Verification items for the finished model (mm, model axes). Face numbers are marked on the shaded views. A direction names the side the tool comes from. Give positions to 0.01 mm unless a question says otherwise; leave off trailing zeros. Loops run counter-clockwise (first coordinate to the right, second up) from the corner with the lowest first, then second, coordinate; pieces in that order, holes last. Notation, with made-up numbers: (68.25, 28) -> (107.25, 28) arc R10 cw to (107.25, 38) -> close; hole circle Ø10 at (-13, 18). An arc over 180 degrees is marked (long way). Answer in a Markdown table with one row per item. Add a question column.
Q1. Release check for a two-part mould opening along Z. For the marked faces 1, 2 and 3 record: pulls with the +Z half, pulls with the -Z half, needs draft (parallel to the pull), parting line crosses it, or undercut.
Q2. Section check D-D on z = -15.5. Enter the section's corners in (x, y).
Q3. Set-up check for the marked faces 4, 5 and 6: record each of +Z, -Z, +X, -X, +Y, -Y from which the full face is reachable in a straight line by a thin tool's end or side.
Q4. Material ranges on probe 1 along X at (y, z) = (7.65, 16); probe 2 along X at (y, z) = (2.5, 16.5), recorded low to high.
Q5. Section check C-C on x = -4. Enter the section's corners in (y, z), and give its area (3 significant figures).
Q6. Section check A-A on y = 8.75. Give the number of separate pieces and of enclosed holes in the cut face, and give its area (3 significant figures).
Q7. Gauge pin test, flat ends, axial feed: P1, Ø0.8, axis at x = 19.5, y = 7.5, coming from the -Z side; P2, Ø0.9, axis at y = 7, z = -15, coming from the -X side; P3, Ø0.8, axis at x = 9.5, y = 2.5, coming from the +Z side. Record the tip position at first contact, or that the pin passes through.
```python
from build123d import *

# Parameters (mm, degrees)
SKETCH1_W           = 40
SKETCH1_H           = 40
BOSS_EXTRUDE1_DEPTH = 5
SKETCH3_R           = 1
BOSS_EXTRUDE3_DEPTH = 5
SKETCH3_4_R         = 1
CUT_EXTRUDE1_DEPTH  = 5
SKETCH4_R           = 1
CUT_EXTRUDE2_DEPTH  = 10
CIRPATTERN2_COUNT   = 4


with BuildPart() as part:
    # Sketch1 → Boss-Extrude1 (new body)
    with BuildSketch(Plane(origin=(0, 0, 0), x_dir=(1, 0, 0), z_dir=(0, 1, 0))):
        Rectangle(SKETCH1_W, SKETCH1_H)
    extrude(amount=BOSS_EXTRUDE1_DEPTH)

    # Sketch3 → Boss-Extrude3 (add)
    # profile 1 of 4: a face of its own
    with BuildSketch(Plane(origin=(0, 5, 0), x_dir=(1, 0, 0), z_dir=(0, 1, 0))):
        with BuildLine():
            Line((11, 11), (18, 11))
            Line((18, 11), (18, 4))
            Line((18, 4), (20, 4))
            Line((20, 4), (20, 13))
            Line((20, 13), (19, 13))
            Line((19, 13), (19, 16))
            ThreePointArc((19, 16), (16, 19), (13, 16))
            Line((13, 16), (13, 13))
            Line((13, 13), (11, 13))
            Line((11, 13), (11, 11))
        make_face()
        with Locations(Location((16, 16, 0), (0, 0, 270))):
            Circle(SKETCH3_R, mode=Mode.SUBTRACT)
    # profile 2 of 4: a face of its own
    with BuildSketch(Plane(origin=(0, 5, 0), x_dir=(1, 0, 0), z_dir=(0, 1, 0))):
        with BuildLine():
            Line((-18, 11), (-11, 11))
            Line((-11, 11), (-11, 13))
            Line((-11, 13), (-13, 13))
            Line((-13, 13), (-13, 16))
            ThreePointArc((-13, 16), (-16, 19), (-19, 16))
            Line((-19, 16), (-19, 13))
            Line((-19, 13), (-20, 13))
            Line((-20, 13), (-20, 9))
            Line((-20, 9), (-18, 9))
            Line((-18, 9), (-18, 11))
        make_face()
        with BuildLine():
            ThreePointArc((-17, 16), (-16, 17), (-15, 16))
            Line((-15, 16), (-17, 16))
        make_face(mode=Mode.SUBTRACT)
    # profile 3 of 4: a face of its own
    with BuildSketch(Plane(origin=(0, 5, 0), x_dir=(1, 0, 0), z_dir=(0, 1, 0))):
        with BuildLine():
            Line((20, -4), (18, -4))
            Line((18, -4), (18, -11))
            Line((18, -11), (11, -11))
            Line((11, -11), (11, -13))
            Line((11, -13), (13, -13))
            Line((13, -13), (13, -16))
            ThreePointArc((13, -16), (16, -19), (19, -16))
            Line((19, -16), (19, -13))
            Line((19, -13), (20, -13))
            Line((20, -13), (20, -4))
        make_face()
    # profile 4 of 4: a face of its own
    with BuildSketch(Plane(origin=(0, 5, 0), x_dir=(1, 0, 0), z_dir=(0, 1, 0))):
        with BuildLine():
            Line((-11, -13), (-11, -11))
            Line((-11, -11), (-18, -11))
            Line((-18, -11), (-18, -9))
            Line((-18, -9), (-20, -9))
            Line((-20, -9), (-20, -13))
            Line((-20, -13), (-19, -13))
            Line((-19, -13), (-19, -16))
            ThreePointArc((-19, -16), (-16, -19), (-13, -16))
            Line((-13, -16), (-13, -13))
            Line((-13, -13), (-11, -13))
        make_face()
        with BuildLine():
            ThreePointArc((-15, -16), (-16, -17), (-17, -16))
            Line((-17, -16), (-15, -16))
        make_face(mode=Mode.SUBTRACT)
    extrude(amount=BOSS_EXTRUDE3_DEPTH)

    # Sketch3_4 → Cut-Extrude1 (cut)
    with BuildSketch(Plane(origin=(0, 5, 0), x_dir=(1, 0, 0), z_dir=(0, 1, 0))):
        with Locations(Location((-16, 16, 0), (0, 0, 270))):
            Circle(SKETCH3_4_R)
        with Locations(Location((-16, -16, 0), (0, 0, 270))):
            Circle(SKETCH3_4_R)
        with Locations(Location((16, -16, 0), (0, 0, 270))):
            Circle(SKETCH3_4_R)
    extrude(amount=CUT_EXTRUDE1_DEPTH, mode=Mode.SUBTRACT)

    # Sketch4 → Cut-Extrude2 (cut)
    with BuildSketch(Plane.ZY.offset(20)):
        with Locations((-10, 2.5)):
            Circle(SKETCH4_R)
        with Locations(Location((10, 2.5, 0), (0, 0, 180))):
            Circle(SKETCH4_R)
    cut_extrude2 = extrude(amount=-CUT_EXTRUDE2_DEPTH, mode=Mode.SUBTRACT)

    # CirPattern2: Cut-Extrude2 ×4 about axis
    cirpattern2_axis = Axis((0, 0, 0), (0, 1, 0))
    for i in range(1, CIRPATTERN2_COUNT):
        add(cut_extrude2.rotate(cirpattern2_axis, i * 360 / CIRPATTERN2_COUNT), mode=Mode.SUBTRACT)


solid = part.part
```
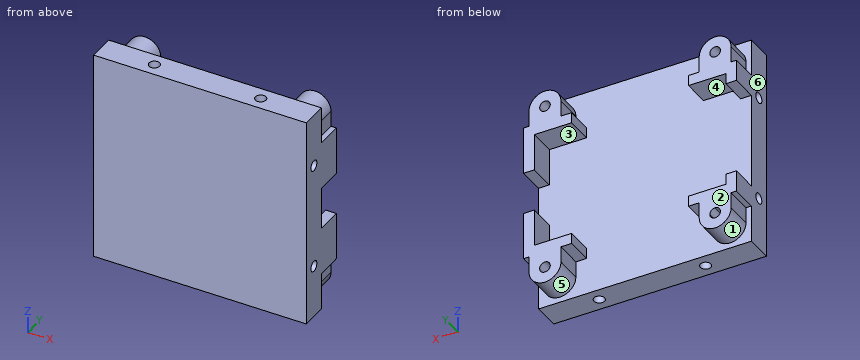
Taken from the geometry:
| question | item | result |
|---|---|---|
| 1 | face 1 | pulls with the -Z half |
| 1 | face 2 | needs draft |
| 1 | face 3 | undercut |
| 2 | outline | (-20, 0) -> (20, 0) -> (20, 5) -> (19, 5) -> (19, 10) -> (16.87, 10) -> (16.87, 5) -> (15.13, 5) -> (15.13, 10) -> (13, 10) -> (13, 5) -> (-13, 5) -> (-13, 10) -> (-15.13, 10) -> (-15.13, 5) -> (-16.87, 5) -> (-16.87, 10) -> (-19, 10) -> (-19, 5) -> (-20, 5) -> close; hole circle Ø2 at (-10, 2.5); hole circle Ø2 at (10, 2.5) |
| 3 | face 4 | +Y |
| 3 | face 5 | -Z, +Y |
| 3 | face 6 | +Z, -Z, -X, +Y, -Y |
| 4 | probe 1 | x = -19 to -17, -15 to -13, 13 to 15, 17 to 19 |
| 4 | probe 2 | x = -20 to -11, -9 to 9, 11 to 20 |
| 5 | outline | (0, -20) -> (5, -20) -> (5, 20) -> (0, 20) -> close |
| 5 | area | 200 mm² |
| 6 | separate pieces | 4 |
| 6 | enclosed holes | 4 |
| 6 | area | 224 mm² |
| 7 | P1 | stops at z = -13 |
| 7 | P2 | stops at x = -19 |
| 7 | P3 | stops at z = 10 |
